Study the drawing (mm; zero at the part's minimum x, y, z) and answer. Round coordinates to 2 decimals unless told otherwise and drop trailing zeros. Loops run counter-clockwise (first coordinate to the right, second up) from the corner with the lowest first, then second, coordinate; pieces in that order, holes last. Notation, with made-up numbers: M -2,59 L 5,59 A12 cw 5,78 Z; hole C 31.25,46 d11. An arc over 180 degrees is marked long. Put each result on its own line as item: value. Start each with the question number.
(1) Section B-B, the plane z = 1.4 is taken. Determine the outline of the cut face in (x, y).
(2) Straight lines are drawn through the part: line 1 (Y direction, x = 13, z = 0.55); line 2 (Y direction, x = 20, z = 0.15); line 3 (Y direction, x = 6, z = 1.3). For each, find the intervals that lie inside material, in ascending order.
(3) Section D-D, the plane y = 19.25 is taken. Determine the outline of the cut face in (x, z).
(4) Flat-ended cylindrical pins translate along their axes: P1, Ø4, axis at x = 20, y = 6, coming from the -Z side; P2, Ø3.5, axis at x = 20, y = 20, coming from the +Z side. Find the tip coordinate at first contact, or state that the pin passes through.
(5) Section A-A, the plane y = 13 is taken. Determine the outline of the cut face in (x, z).
(6) Determine the mould class of the marked faces 1, 2 and 3 for opening direction Y: released by +Y, released by -Y, zero draft, split by the parting line, or undercut.
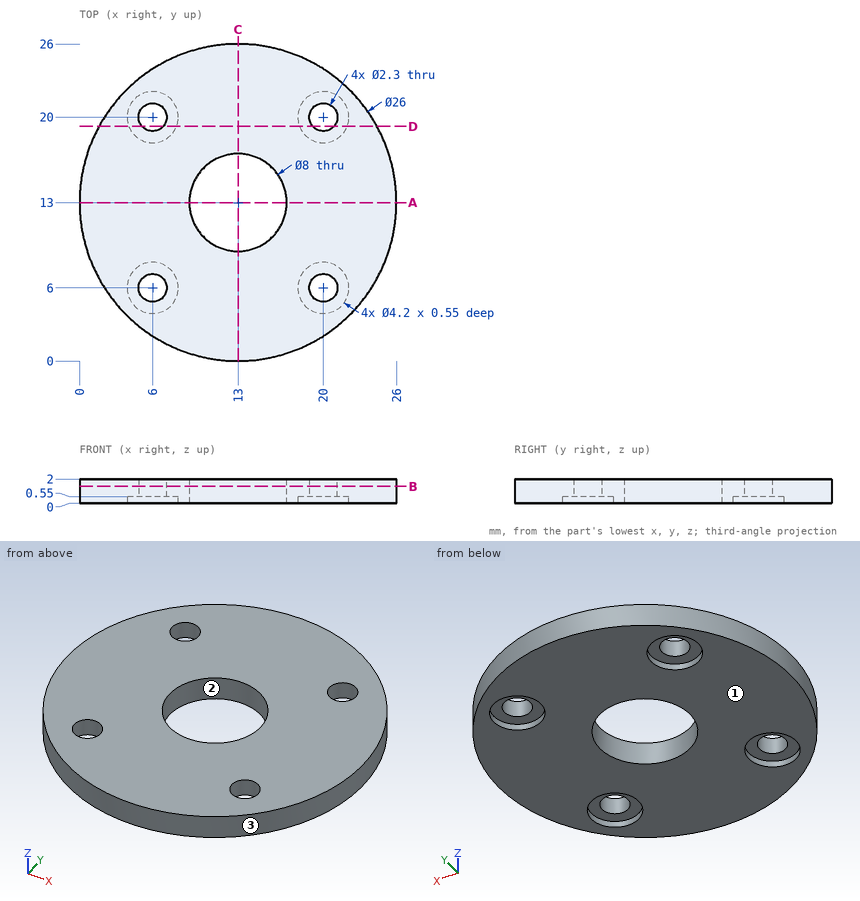
Recorded:
1. outline: C 13,13 d26; hole C 6,6 d2.3; hole C 6,20 d2.3; hole C 13,13 d8; hole C 20,6 d2.3; hole C 20,20 d2.3
2. line 1: y = 0 to 9, 17 to 26
2. line 2: y = 2.05 to 3.9, 8.1 to 17.9, 22.1 to 23.95
2. line 3: y = 2.05 to 4.85, 7.15 to 18.85, 21.15 to 23.95
3. outline: M 1.6,0 L 4.04,0 L 4.04,0.55 L 5.13,0.55 L 5.13,2 L 1.6,2 Z; M 6.87,0.55 L 7.96,0.55 L 7.96,0 L 18.04,0 L 18.04,0.55 L 19.13,0.55 L 19.13,2 L 6.87,2 Z; M 20.87,0.55 L 21.96,0.55 L 21.96,0 L 24.4,0 L 24.4,2 L 20.87,2 Z
4. P1: stops at z = 0.55
4. P2: stops at z = 2
5. outline: M 0,0 L 9,0 L 9,2 L 0,2 Z; M 17,0 L 26,0 L 26,2 L 17,2 Z
6. face 1: zero draft
6. face 2: undercut
6. face 3: split by the parting line
